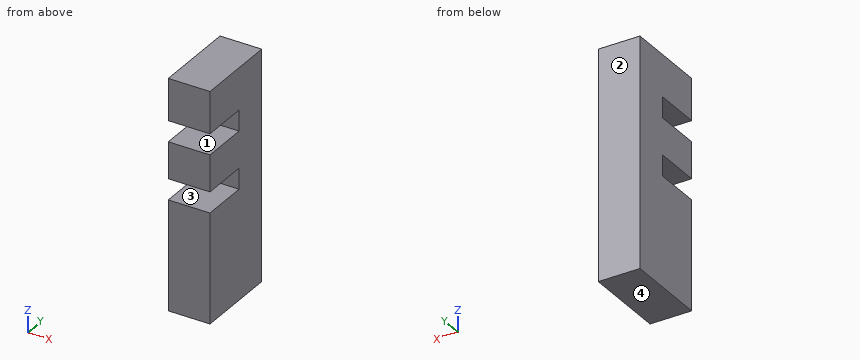
Autodesk Inventor part; units mm, degrees
ref_plane "YZ Plane" through (0, 0, 0) normal (1, 0, 0) x (0, 1, 0)
ref_plane "XZ Plane" through (0, 0, 0) normal (0, 1, 0) x (-1, 0, 0)
ref_plane "XY Plane" through (0, 0, 0) normal (0, 0, 1) x (1, 0, 0)
sketch "Sketch1" plane through (0, 0, 0) normal (0, 0, 1) x (1, 0, 0)
  line L0 (0, 0) -> (50.8, 0)
  line L1 (50.8, 0) -> (50.8, 101.6)
  line L2 (50.8, 101.6) -> (0, 101.6)
  line L3 (0, 101.6) -> (0, 0)
  dimension "d0" = 50.8
  dimension "d1" = 101.6
extrude "Extrusion1" add sketch "Sketch1" along normal blind 279.4
sketch "Sketch2" plane through (50.8, 0, 0) normal (1, 0, 0) x (0, 0, -1)
  line L0 (0, 0) -> (-279.4, 0)
  line L1 (-228.6, 0) -> (-203.2, 0)
  line L2 (-203.2, 0) -> (-203.2, 57.15)
  line L3 (-203.2, 57.15) -> (-228.6, 57.15)
  line L4 (-228.6, 57.15) -> (-228.6, 0)
  line L5 (-279.4, 0) -> (-279.4, 101.6)
  line L6 (-158.75, 0) -> (-133.35, 0)
  line L7 (-133.35, 0) -> (-133.35, 57.15)
  line L8 (-133.35, 57.15) -> (-158.75, 57.15)
  line L9 (-158.75, 57.15) -> (-158.75, 0)
  dimension "d4" = 25.4
  dimension "d5" = 57.15
  dimension "d6" = 50.8
  dimension "d7" = 25.4
  dimension "d8" = 44.45
extrude "Extrusion2" cut sketch "Sketch2" against normal blind 266.7
properties part number "LargeSideHook"
Part model, mm, in its own coordinate system. Face numbers are marked on the shaded views. Coordinates: 2 decimals unless noted, no trailing zeros. Order: outer loops, then holes, each group sorted by start corner. A loop starts at its lowest first (then second) coordinate and runs counter-clockwise, first axis right, second up. Notation, with made-up numbers: M 13,68 L 30,68 A11 cw 30,80 Z; hole C -8.75,71.25 d11. An arc over 180 degrees is marked long. Use a Markdown table: item, result.
(1) Probe L1, parallel to Z at x = 39, y = 53. List the from-to ranges inside material, lowest first.
A:
| item | result |
|---|---|
| L1 | z = 0 to 133.35, 158.75 to 203.2, 228.6 to 279.4 |
(2) Cut at B-B on x = 46. Write the cut outline in (y, z), then the cut area to 3 significant figures.
A:
| item | result |
|---|---|
| outline | M 0,0 L 101.6,0 L 101.6,279.4 L 0,279.4 L 0,228.6 L 57.15,228.6 L 57.15,203.2 L 0,203.2 L 0,158.75 L 57.15,158.75 L 57.15,133.35 L 0,133.35 Z |
| area | 25,500 mm^2 |
(3) Flat gauge pins, fed straight in: pin 1 (6 mm diameter, centred on y = 64, z = 62.5, fed in from -X); pin 2 (7.5 mm diameter, centred on x = 14, z = 150, fed in from -Y). Where does each tip first touch, or does it go through?
A:
| item | result |
|---|---|
| pin 1 | stops at x = 0 |
| pin 2 | stops at y = 57.15 |
(4) Cut at A-A on y = 11. Write the cut outline in (x, z).
A:
| item | result |
|---|---|
| outline | M 0,0 L 50.8,0 L 50.8,133.35 L 0,133.35 Z; M 0,158.75 L 50.8,158.75 L 50.8,203.2 L 0,203.2 Z; M 0,228.6 L 50.8,228.6 L 50.8,279.4 L 0,279.4 Z |
(5) Cut at C-C on z = 148. Write the cut outline in (x, y), then the cut area to 3 significant figures.
A:
| item | result |
|---|---|
| outline | M 0,57.15 L 50.8,57.15 L 50.8,101.6 L 0,101.6 Z |
| area | 2,260 mm^2 |
(6) Pull direction Z, two halves, no side cores. Call the marked faces 1, 2, 3 and 4: released by +Z, released by -Z, zero draft, split by the parting line, or undercut.
A:
| item | result |
|---|---|
| face 1 | undercut |
| face 2 | zero draft |
| face 3 | undercut |
| face 4 | released by -Z |
